from build123d import *

# Parameters (mm, degrees)
SKETCH1_R               = 30
SKETCH1_R_2             = 20
BOSS_EXTRUDE1_DEPTH     = 10
SKETCH2_OUTSIDE_W       = 79.436
SKETCH2_OUTSIDE_H       = 79.436
SKETCH2_OUTSIDE_R       = 20
CUT_EXTRUDE1_DEPTH      = 3.5
CUT_EXTRUDE3_DEPTH      = 47.904157598
CUT_EXTRUDE3_DEPTH_BACK = 47.904157598
SKETCH4_R               = 2.6
SKETCH5_R               = 30
SKETCH5_R_2             = 20
CUT_EXTRUDE4_DEPTH      = 3


with BuildPart() as part:
    # Sketch1 → Boss-Extrude1 (new, symmetric)
    # profile 1 of 2: a face of its own
    with BuildSketch(Plane.XY):
        Circle(SKETCH1_R)
        Circle(SKETCH1_R_2, mode=Mode.SUBTRACT)
    # profile 2 of 2: a face of its own
    with BuildSketch(Plane.XY):
        Circle(SKETCH1_R_2)
    extrude(amount=BOSS_EXTRUDE1_DEPTH, both=True)

    # Sketch2 outside → Cut-Extrude1 (cut, symmetric)
    with BuildSketch(Plane.XY.offset(5)):
        Rectangle(SKETCH2_OUTSIDE_W, SKETCH2_OUTSIDE_H)
        Circle(SKETCH2_OUTSIDE_R, mode=Mode.SUBTRACT)
    cut_extrude1 = extrude(amount=CUT_EXTRUDE1_DEPTH, both=True, mode=Mode.SUBTRACT)

    # Mirror1: Cut-Extrude1 across plane
    add(cut_extrude1.mirror(Plane.XY), mode=Mode.SUBTRACT)

    # Sketch4 → Cut-Extrude3 (cut, two sides: drawn at the far end of the back side and taken through both)
    with BuildSketch(Plane(origin=(0, 0, -10), x_dir=(-1, 0, 0), z_dir=(0, 0, -1)).offset(-CUT_EXTRUDE3_DEPTH_BACK)):
        Circle(SKETCH4_R)
    extrude(amount=CUT_EXTRUDE3_DEPTH + CUT_EXTRUDE3_DEPTH_BACK, mode=Mode.SUBTRACT)

    # Sketch5 → Cut-Extrude4 (cut)
    with BuildSketch(Plane.XY.offset(1.5)):
        Circle(SKETCH5_R)
        Circle(SKETCH5_R_2, mode=Mode.SUBTRACT)
    extrude(amount=-CUT_EXTRUDE4_DEPTH, mode=Mode.SUBTRACT)


solid = part.part
The model under review builds one solid part; all positions refer to its coordinate system, in mm. A direction names the side the tool comes from. Round coordinates to 2 decimals unless told otherwise and drop trailing zeros. Loops run counter-clockwise (first coordinate to the right, second up) from the corner with the lowest first, then second, coordinate; pieces in that order, holes last. Notation, with made-up numbers: M 32.5,-35 L 60.5,-35 A25 cw 60.5,-23 Z; hole C 32.25,58 d6. An arc over 180 degrees is marked long. Answer as CSV lines item,"result". Start each with the question number.
Item 1: Insertion check: P1, Ø1.5, axis at x = 13.5, z = -1, coming from the -Y side; P2, Ø10, axis at x = 21.5, z = -3, coming from the +Y side; P3, Ø8, axis at x = 7, z = 3, coming from the -Y side. Each pin has a flat end and moves straight along its axis. Give the tip position at first contact, or say it passes through.
Item 2: Wall thickness on line 1 (Y direction, x = 0, z = -0.5); line 2 (Z direction, x = -16, y = -13); line 3 (Y direction, x = 15, z = 8.25): over which ranges is each line inside the solid? List them lowest first. Write a range as [from, to].
Item 3: Mouldability with a two-part tool opening along X and no side actions: class faces 3 (the face through (6, 0, 10)), 4 (the face through (-29.97, 1.32, 9.26)), 5 (the face through (0.338, 2.578, 0.14)) as released by +X, released by -X, zero draft, split by the parting line, or undercut.
Item 4: Consider section C-C (y = -24). Write out the cut boundary in (x, z).
Item 5: For faces 1 (the face through (6, -20, 8.5)), 2 (the face through (0, -6, -10)), list the 3-axis set-ups (+Z, -Z, +X, -X, +Y, -Y) from which the entire face can be reached by the end or side of a thin tool; tool diameter is ignored.
Item 6: Consider section A-A (y = 0). Write out the cut boundary in (x, z), then the cut area to 3 significant figures.
Item 7: Consider section D-D (z = -0.75). Write out the cut boundary in (x, y), then the cut area to 3 significant figures.
Answer:
1,P1,"stops at y = -15.41"
1,P2,"stops at y = 11.3"
1,P3,"stops at y = -19.77"
2,line 1,"y = [-20, -2.6], [2.6, 20]"
2,line 2,"z = [-10, -8.5], [8.5, 10]"
2,line 3,"y = [-13.23, 13.23]"
3,face 3,"zero draft"
3,face 4,"split by the parting line"
3,face 5,"undercut"
4,outline,"M -18,-10 L 18,-10 L 18,-8.5 L -18,-8.5 Z; M -18,8.5 L 18,8.5 L 18,10 L -18,10 Z"
5,face 1,"none"
5,face 2,"-Z, +X, -X, +Y, -Y"
6,outline,"M -30,-10 L -2.6,-10 L -2.6,10 L -30,10 L -30,8.5 L -20,8.5 L -20,-8.5 L -30,-8.5 Z; M 2.6,-10 L 30,-10 L 30,-8.5 L 20,-8.5 L 20,8.5 L 30,8.5 L 30,10 L 2.6,10 Z"
6,area,"756 mm^2"
7,outline,"C 0,0 d40; hole C 0,0 d5.2"
7,area,"1,240 mm^2"
